```python
from build123d import *

# Parameters (mm, degrees)
BOSS_EXTRUDE5_DEPTH = 390
SKETCH7_R           = 30
CUT_EXTRUDE4_DEPTH  = 120
SKETCH10_W          = 110
SKETCH10_H          = 140
CUT_EXTRUDE6_DEPTH  = 841.059521701
CUT_EXTRUDE9_START  = -390
SKETCH13_W          = 30
SKETCH13_H          = 110
CUT_EXTRUDE9_DEPTH  = 390
SKETCH15_W          = 60
SKETCH15_H          = 60
CUT_EXTRUDE10_DEPTH = 470


with BuildPart() as part:
    # Sketch1 → Boss-Extrude5 (new body)
    with BuildSketch(Plane(origin=(0, 0, 0), x_dir=(1, 0, 0), z_dir=(0, 1, 0))):
        Polygon((0, 0), (440, 0), (440, 150), (100, 150), (100, 600), (0, 600), align=None)
    extrude(amount=BOSS_EXTRUDE5_DEPTH)

    # Sketch7 → Cut-Extrude4 (cut)
    with BuildSketch(Plane(origin=(0, 0, -150), x_dir=(-1, 0, 0), z_dir=(0, 0, -1))):
        with Locations((-190, 250)):
            Circle(SKETCH7_R)
    extrude(amount=-CUT_EXTRUDE4_DEPTH, mode=Mode.SUBTRACT)

    # Sketch10 → Cut-Extrude6 (cut, through all)
    with BuildSketch(Plane(origin=(440, 0, 0), x_dir=(0, 0, -1), z_dir=(1, 0, 0))):
        with Locations((75, 250)):
            Rectangle(SKETCH10_W, SKETCH10_H)
    extrude(amount=-CUT_EXTRUDE6_DEPTH, mode=Mode.SUBTRACT)

    # Sketch13 → Cut-Extrude9 (cut)
    with BuildSketch(Plane.XZ.offset(CUT_EXTRUDE9_START)):
        with Locations((65, -75)):
            Rectangle(SKETCH13_W, SKETCH13_H)
        with Locations((35, -75)):
            Rectangle(SKETCH13_W, SKETCH13_H)
    extrude(amount=CUT_EXTRUDE9_DEPTH, mode=Mode.SUBTRACT)

    # Sketch15 → Cut-Extrude10 (cut)
    with BuildSketch(Plane(origin=(0, 0, -600), x_dir=(-1, 0, 0), z_dir=(0, 0, -1))):
        with Locations((-50, 250)):
            Rectangle(SKETCH15_W, SKETCH15_H)
    extrude(amount=-CUT_EXTRUDE10_DEPTH, mode=Mode.SUBTRACT)


solid = part.part
```
Check sheet for the modelled part. Datum: model origin and axes. Units: mm. A direction names the side the tool comes from. Coordinates: 2 decimals unless noted, no trailing zeros. Write each loop counter-clockwise with the first axis right and the second up, starting at its lowest first coordinate (ties: lowest second). Pieces come first, ordered by that corner, then holes. Notation, with made-up numbers: M -37.75,18.5 L -31.75,18.5 A29 cw -31.75,57.5 Z; hole C 52,-18.5 d10. An arc over 180 degrees is marked long. Use one line per item in the form item = value.
Item 1: Release check for a two-part mould opening along Z. For faces 1 (the face through (80, 355, -76)), 2 (the face through (217, 192, 0)), 3 (the face through (272, 192, -150)), 4 (the face through (100, 192, -372)) record: pulls with the +Z half, pulls with the -Z half, needs draft (parallel to the pull), parting line crosses it, or undercut.
Answer below:
face_1 = undercut
face_2 = pulls with the +Z half
face_3 = pulls with the -Z half
face_4 = needs draft
Item 2: Sectioned sample at A-A, the plane z = -78. Record the cut outline in (x, y).
Answer below:
outline = M 0,0 L 20,0 L 20,180 L 0,180 Z; M 0,320 L 20,320 L 20,390 L 0,390 Z; M 80,0 L 440,0 L 440,180 L 80,180 Z; M 80,320 L 440,320 L 440,390 L 80,390 Z
Item 3: Sectioned sample at D-D, the plane z = -205.5. Record the cut outline in (x, y).
Answer below:
outline = M 0,0 L 100,0 L 100,390 L 0,390 Z; hole M 20,220 L 80,220 L 80,280 L 20,280 Z
Item 4: Material ranges on L1, parallel to X at y = 270, z = -570; L2, parallel to Y at x = 190, z = -138.25; L3, parallel to Z at x = 204.5, y = 315, recorded low to high. Write a range as from..to.
Answer below:
L1 = 0..20, 80..100
L2 = 0..220, 280..390
L3 = -150..-130, -20..0
Item 5: Sectioned sample at C-C, the plane y = 110.5. Record the cut outline in (x, z), and give its area (3 significant figures).
Answer below:
outline = M 0,-600 L 100,-600 L 100,-150 L 440,-150 L 440,0 L 0,0 Z; hole M 20,-130 L 80,-130 L 80,-20 L 20,-20 Z
area = 104,000 mm^2
Item 6: Sectioned sample at B-B, the plane y = 250. Record the cut outline in (x, z).
Answer below:
outline = M 0,-600 L 20,-600 L 20,-130 L 0,-130 Z; M 0,-20 L 440,-20 L 440,0 L 0,0 Z; M 80,-600 L 100,-600 L 100,-150 L 160,-150 L 160,-130 L 80,-130 Z; M 220,-150 L 440,-150 L 440,-130 L 220,-130 Z
Item 7: Set-up check for faces 5 (the face through (10, 180, -74)), 6 (the face through (50, 220, -368)), 7 (the face through (20, 355, -76)), 8 (the face through (174, 236, -20)): record each of +Z, -Z, +X, -X, +Y, -Y from which the full face is reachable in a straight line by a thin tool's end or side.
Answer below:
face_5 = +X, -X
face_6 = -Z
face_7 = +Y, -Y
face_8 = none
Item 8: Gauge pin test, flat ends, axial feed: pin 1 Ø8 at (y, z) = (347, -404) entering from +X; pin 2 Ø3 at (x, y) = (336.5, 350.5) entering from -Z. Record the tip position at first contact, or that the pin passes through.
Answer below:
pin_1 = 100
pin_2 = -150
